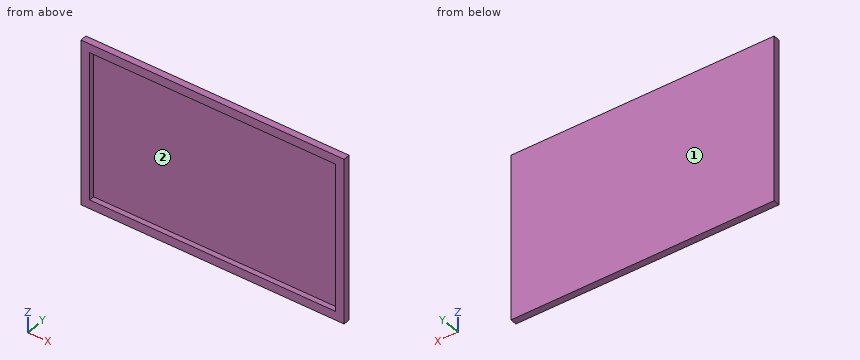
from build123d import *

# Parameters (mm, degrees)
SKETCH1_W           = 1502
SKETCH1_H           = 946
BOSS_EXTRUDE1_DEPTH = 38
SKETCH1_4_W         = 1402
SKETCH1_4_H         = 846
CUT_EXTRUDE1_DEPTH  = 30


with BuildPart() as part:
    # Sketch1 → Boss-Extrude1 (new body)
    with BuildSketch(Plane(origin=(0, 0, 0), x_dir=(1, 0, 0), z_dir=(0, 1, 0))):
        with Locations((167.925465839, -6.540372671)):
            Rectangle(SKETCH1_W, SKETCH1_H)
    extrude(amount=BOSS_EXTRUDE1_DEPTH)

    # Sketch1<4> → Cut-Extrude1 (cut)
    with BuildSketch(Plane(origin=(0, 0, 0), x_dir=(1, 0, 0), z_dir=(0, 1, 0))):
        with Locations((167.925465839, -6.540372671)):
            Rectangle(SKETCH1_4_W, SKETCH1_4_H)
    extrude(amount=CUT_EXTRUDE1_DEPTH, mode=Mode.SUBTRACT)


solid = part.part
Here's how the part is built. I have some questions about the finished solid (model axes, mm). Face numbers are marked on the shaded views. Coordinates: 2 decimals unless noted, no trailing zeros. Order: outer loops, then holes, each group sorted by start corner. A loop starts at its lowest first (then second) coordinate and runs counter-clockwise, first axis right, second up. Notation, with made-up numbers: M -4,-2.5 L 42,-2.5 A33 cw 42,33.5 Z; hole C -14.75,-32 d11. An arc over 180 degrees is marked long. Answer as CSV lines item,"result". Start each with the question number.
1. I need wall thicknesses on line 1 (X direction, y = 23, z = 98.5); line 2 (Z direction, x = 762.5, y = 27); line 3 (Y direction, x = -187, z = 305). Which ranges of each line are inside material? Lowest first, please. Write a range as [from, to].
2. I want a section at A-A, the plane z = 1. Write out the boundary of the cut face in (x, y).
3. We'd pull the mould along Z, two halves only. Please class the marked faces 1 and 2: released by +Z, released by -Z, zero draft, split by the parting line, or undercut.
4. I want a section at C-C, the plane x = -167.5. Write out the boundary of the cut face in (y, z).
5. I want a section at B-B, the plane y = 22.5. Write out the boundary of the cut face in (x, z), and give its area (3 significant figures).
Recorded:
1,line 1,"x = [-583.07, -533.07], [868.93, 918.93]"
1,line 2,"z = [-466.46, -416.46], [429.54, 479.54]"
1,line 3,"y = [30, 38]"
2,outline,"M -583.07,0 L -533.07,0 L -533.07,30 L 868.93,30 L 868.93,0 L 918.93,0 L 918.93,38 L -583.07,38 Z"
3,face 1,"zero draft"
3,face 2,"undercut"
4,outline,"M 0,-466.46 L 38,-466.46 L 38,479.54 L 0,479.54 L 0,429.54 L 30,429.54 L 30,-416.46 L 0,-416.46 Z"
5,outline,"M -583.07,-466.46 L 918.93,-466.46 L 918.93,479.54 L -583.07,479.54 Z; hole M -533.07,-416.46 L 868.93,-416.46 L 868.93,429.54 L -533.07,429.54 Z"
5,area,"235,000 mm2"
